Can you work these out from the drawing? Everything is in mm from the part's minimum corner. Round coordinates to 2 decimals unless told otherwise and drop trailing zeros. Write each loop counter-clockwise with the first axis right and the second up, starting at its lowest first coordinate (ties: lowest second). Pieces come first, ordered by that corner, then holes.
Q1. Please list where these lines run through material, in increasing order: line 1 along X through (y, z) = (1.35, 30); line 2 along Z through (x, y) = (75, 0.4); line 3 along X through (y, z) = (1.1, 2.5).
Q2. If we section it at D-D (z = 2.5): Please give me the cut outline in (x, y), plus the area to 3 significant figures.
Q3. If we section it at B-B (z = 35): Please give me the cut outline in (x, y).
Q4. If we section it at C-C (x = 102.5): Please give me the cut outline in (y, z).
Q5. If we section it at A-A (x = 7.5): Please give me the cut outline in (y, z), plus the area to 3 significant figures.
Q6. I'm going to push a flat-ended pin straight in: pin 1 Ø2 at (x, z) = (7.5, 2.5) entering from -Y. Where does the tip first touch, or does it pass through?
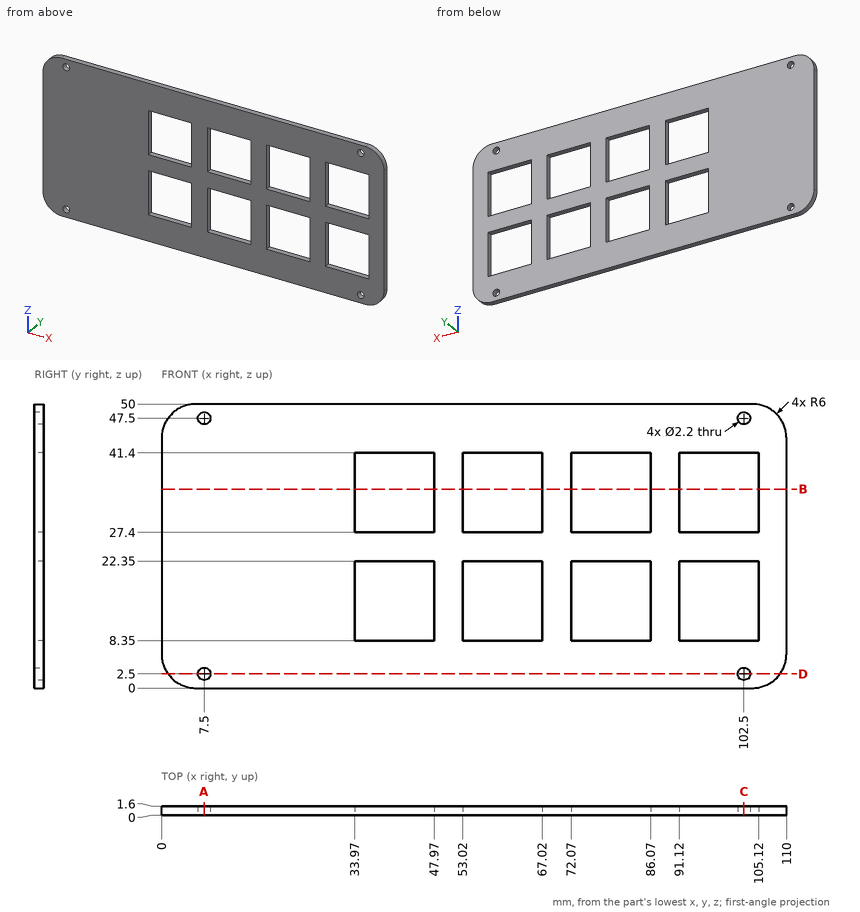
A:
1. line 1: x = 0 to 33.97, 47.97 to 53.02, 67.02 to 72.07, 86.07 to 91.12, 105.12 to 110
1. line 2: z = 0 to 8.35, 22.35 to 27.4, 41.4 to 50
1. line 3: x = 1.13 to 6.4, 8.6 to 101.4, 103.6 to 108.87
2. outline: (1.13, 0) - (6.4, 0) - (6.4, 1.6) - (1.13, 1.6) - close; (8.6, 0) - (101.4, 0) - (101.4, 1.6) - (8.6, 1.6) - close; (103.6, 0) - (108.87, 0) - (108.87, 1.6) - (103.6, 1.6) - close
2. area: 165 mm2
3. outline: (0, 0) - (33.97, 0) - (33.97, 1.6) - (0, 1.6) - close; (47.97, 0) - (53.02, 0) - (53.02, 1.6) - (47.97, 1.6) - close; (67.02, 0) - (72.07, 0) - (72.07, 1.6) - (67.02, 1.6) - close; (86.07, 0) - (91.12, 0) - (91.12, 1.6) - (86.07, 1.6) - close; (105.12, 0) - (110, 0) - (110, 1.6) - (105.12, 1.6) - close
4. outline: (0, 0) - (1.6, 0) - (1.6, 1.4) - (0, 1.4) - close; (0, 3.6) - (1.6, 3.6) - (1.6, 8.35) - (0, 8.35) - close; (0, 22.35) - (1.6, 22.35) - (1.6, 27.4) - (0, 27.4) - close; (0, 41.4) - (1.6, 41.4) - (1.6, 46.4) - (0, 46.4) - close; (0, 48.6) - (1.6, 48.6) - (1.6, 50) - (0, 50) - close
5. outline: (0, 0) - (1.6, 0) - (1.6, 1.4) - (0, 1.4) - close; (0, 3.6) - (1.6, 3.6) - (1.6, 46.4) - (0, 46.4) - close; (0, 48.6) - (1.6, 48.6) - (1.6, 50) - (0, 50) - close
5. area: 73.0 mm2
6. pin 1: passes through
